```python
from build123d import *

# Parameters (mm, degrees)
SKETCH1_R                    = 1
EXTRUDE1_DEPTH               = 4
SKETCH1_3_R                  = 2.38125
EXTRUDE4_DEPTH               = 2
M2X0_4_TAPPED_HOLE1_D        = 1.6
M2X0_4_TAPPED_HOLE1_DEPTH    = 3
M2X0_4_TAPPED_HOLE1_TIP      = 0.480688495
F_2_0_2_DIAMETER_HOLE1_D     = 2
F_2_0_2_DIAMETER_HOLE1_DEPTH = 10
F_2_0_2_DIAMETER_HOLE1_TIP   = 0.600860619
F_0_80_TAPPED_HOLE2_D        = 1.19126
F_0_80_TAPPED_HOLE2_DEPTH    = 4


with BuildPart() as part:
    # Sketch1 → Extrude1 (new body)
    with BuildSketch(Plane(origin=(0, 0, 0), x_dir=(1, 0, 0), z_dir=(0, 1, 0))):
        with BuildLine():
            Line((-5.186041147, 3.316192399), (2.637731834, -10.234979911))
            ThreePointArc((2.637731834, -10.234979911), (4.802795343, -11.484979911), (6.967858853, -10.234979911))
            Line((6.967858853, -10.234979911), (14.791631834, 3.316192399))
            ThreePointArc((14.791631834, 3.316192399), (14.791631834, 5.816192399), (12.626568324, 7.066192399))
            Line((12.626568324, 7.066192399), (-3.020977638, 7.066192399))
            ThreePointArc((-3.020977638, 7.066192399), (-5.186041147, 5.816192399), (-5.186041147, 3.316192399))
        make_face()
        with Locations((-2.110635714, 4.040606244)):
            Circle(SKETCH1_R, mode=Mode.SUBTRACT)
        with Locations((11.7162264, 4.040606244)):
            Circle(SKETCH1_R, mode=Mode.SUBTRACT)
        with Locations((4.802795343, -7.933807601)):
            Circle(SKETCH1_R, mode=Mode.SUBTRACT)
    extrude(amount=EXTRUDE1_DEPTH)

    # Sketch1<3> → Extrude4 (cut)
    with BuildSketch(Plane(origin=(0, 0, 0), x_dir=(1, 0, 0), z_dir=(0, 1, 0))):
        with Locations((4.802795343, -7.933807601)):
            Circle(SKETCH1_3_R)
        with Locations((11.7162264, 4.040606244)):
            Circle(SKETCH1_3_R)
        with Locations((-2.110635714, 4.040606244)):
            Circle(SKETCH1_3_R)
    extrude(amount=EXTRUDE4_DEPTH, mode=Mode.SUBTRACT)

    # M2x0.4 Tapped Hole1
    with Locations(Plane(origin=(4.802795343, 0, -0.049134963), x_dir=(0, 0, -1), z_dir=(0, -1, 0))):
        with Locations((0, 0)):
            Hole(M2X0_4_TAPPED_HOLE1_D / 2, depth=M2X0_4_TAPPED_HOLE1_DEPTH)
            with Locations((0, 0, -(M2X0_4_TAPPED_HOLE1_DEPTH + M2X0_4_TAPPED_HOLE1_TIP / 2))):  # 118° drill point
                Cone(0, M2X0_4_TAPPED_HOLE1_D / 2, M2X0_4_TAPPED_HOLE1_TIP, mode=Mode.SUBTRACT)

    # Ø2.0 (2) Diameter Hole1
    with Locations(Plane(origin=(4.802795343, 0, -5.066192399), x_dir=(0, 0, -1), z_dir=(0, -1, 0))):
        with Locations((0, 0), (-5.02, 5), (-5.02, -5)):
            Hole(F_2_0_2_DIAMETER_HOLE1_D / 2, depth=F_2_0_2_DIAMETER_HOLE1_DEPTH)
            with Locations((0, 0, -(F_2_0_2_DIAMETER_HOLE1_DEPTH + F_2_0_2_DIAMETER_HOLE1_TIP / 2))):  # 118° drill point
                Cone(0, F_2_0_2_DIAMETER_HOLE1_D / 2, F_2_0_2_DIAMETER_HOLE1_TIP, mode=Mode.SUBTRACT)

    # #0-80 Tapped Hole2
    with Locations(Plane(origin=(1.802795343, 4, -4.036192399), x_dir=(0, 0, 1), z_dir=(0, 1, 0))):
        with Locations((0, 0), (0, 6)):
            Hole(F_0_80_TAPPED_HOLE2_D / 2, depth=F_0_80_TAPPED_HOLE2_DEPTH)


solid = part.part
```
Here's how the part is built. I have some questions about the finished solid (model axes, mm). A direction names the side the tool comes from. Give positions to 0.01 mm unless a question says otherwise; leave off trailing zeros. Loops run counter-clockwise (first coordinate to the right, second up) from the corner with the lowest first, then second, coordinate; pieces in that order, holes last. Notation, with made-up numbers: M 81,59 L 88,59 A32 ccw 88,96 Z; hole C 3.25,63.5 d6. An arc over 180 degrees is marked long. Put each result on its own line as item: value. Start each with the question number.
(1) For faces 1 (the flat face through (5, 4, 0)), 2 (the flat face through (-1.6, 2, -3)), which set-ups out of +Z, -Z, +X, -X, +Y, -Y let a thin tool reach every point of the face, with its end or its side?
(2) I want a section at A-A on x = -2.5. Please give me the cut outline in (y, z).
(3) I need wall thicknesses on line 1 along X through (y, z) = (1.8, -2.25); line 2 along X through (y, z) = (1.6, -0.5); line 3 along Z through (x, y) = (4.5, 2.8). Which ranges of each line are inside material? Lowest first, please. Write a range as [from, to].
(4) I want a section at B-B on z = -5.5. Please give me the cut outline in (x, y), then the cut area to 3 significant figures.
(5) I want a section at D-D on z = 6.25. Please give me the cut outline in (x, y).
(6) Will these pins go through, and if not, where does the flat tip stop? pin 1 Ø1 at (x, y) = (6, 3) entering from +Z; pin 2 Ø1.6 at (x, z) = (-0.2, -0.05) entering from +Y; pin 3 Ø1 at (x, y) = (5.5, 0.5) entering from +Z; pin 4 Ø2.5 at (x, z) = (12, -3.5) entering from -Y.
(7) If we mould it in two halves opening along Z, with no side actions, what happens to faces 3 (the cylindrical face through (-5.167, 1.972, -5.848)), 4 (the flat face through (10.8, 2, 3.6)), 5 (the cylindrical face through (9.337, 0.986, -4.145))? For each: +Z half, -Z half, draft (parallel to the pull), parting line (faces both ways), or undercut.
(8) I want a section at C-C on y = 0.3. State how many separate pieces and enclosed holes the cut face has, then the cut area to 3 significant figures.
Answer block:
1. face 1: +Z, -Z, +X, -X, +Y
1. face 2: -Y
2. outline: M 0,-7.07 L 4,-7.07 L 4,-4.96 L 2,-4.96 L 2,-6.39 L 0,-6.39 Z; M 0,-1.69 L 2,-1.69 L 2,-3.12 L 4,-3.12 L 4,1.34 L 0,1.34 Z
3. line 1: [-4.57, -3.68], [-0.54, 10.15], [13.29, 14.18]
3. line 2: [-3.56, -1.09], [0.69, 4.14], [5.46, 8.91], [10.69, 13.17]
3. line 3: [-7.07, -6.02], [-4.11, -0.79], [0.69, 6.98], [8.89, 11.47]
4. outline: M -5.34,0 L -3.99,0 L -3.99,2 L -0.23,2 L -0.23,0 L 3.9,0 L 3.9,4 L -5.34,4 Z; M 5.7,0 L 9.83,0 L 9.83,2 L 13.6,2 L 13.6,0 L 14.95,0 L 14.95,4 L 5.7,4 Z
4. area: 58.9 mm^2
5. outline: M 0.34,0 L 3.12,0 L 3.12,2 L 6.49,2 L 6.49,0 L 9.27,0 L 9.27,4 L 0.34,4 Z
6. pin 1: z = 11.39
6. pin 2: through
6. pin 3: z = 11.48
6. pin 4: y = 2
7. face 3: parting line
7. face 4: +Z half
7. face 5: undercut
8. separate pieces: 1
8. enclosed holes: 9
8. area: 176 mm^2
